Model file for the job. Use its own axes, mm. A direction names the side the tool comes from. Give positions to 0.01 mm unless a question says otherwise; leave off trailing zeros. Loops run counter-clockwise (first coordinate to the right, second up) from the corner with the lowest first, then second, coordinate; pieces in that order, holes last. Notation, with made-up numbers: M 1,-23.75 L 48,-23.75 A6 ccw 48,-12.75 Z; hole C 53.5,6.5 d3. An arc over 180 degrees is marked long. Use CSV: the item, a comma, the result in double quotes. Start each with the question number.
(1) Two-plate mould, pull along Y, no slides. Class faces 1 (the face through (8, 5.862, 0)), 2 (the face through (10.877, 10.2, 2.5)), 3 (the face through (3, 20, 3)), 4 (the face through (4, 10, -8.672)): pulls with the +Y half, pulls with the -Y half, needs draft (parallel to the pull), parting line crosses it, or undercut.
(2) Slice it at D-D on z = 34. List the corners of the cut face in (x, y), and give its area (3 significant figures).
(3) Flat gauge pins, fed straight in: P1, Ø0.6, axis at x = 3, z = 0, coming from the +Y side; P2, Ø5, axis at x = 7, y = 13.5, coming from the -Z side; P3, Ø9.5, axis at x = -7.5, z = 6, coming from the +Y side; P4, Ø6, axis at y = -3, z = 40, coming from the -X side. Where does each tip first touch, or does it go through?
(4) Slice it at C-C on z = -29. List the corners of the cut face in (x, y), and give its area (3 significant figures).
(5) Tool access for faces 5 (the face through (-3.4, 13.3, -0.1)), 6 (the face through (4, 10, 9.332)), 7 (the face through (8, 14.614, 0)): list every direction of +Z, -Z, +X, -X, +Y, -Y with a clear straight run to the whole face (end or side of a thin tool).
(6) Slice it at B-B on x = 0. List the corners of the cut face in (y, z).
(7) Wall check: line 1 along Z through (x, y) = (0, -7.5); line 2 along Z through (x, y) = (0, 16); line 3 along Y through (x, z) = (3, 0). Give the ranges that are in metal, low to high. Write a range as from..to.
(8) Slice it at A-A on y = -14.5. List the corners of the cut face in (x, z), and give its area (3 significant figures).
```python
from build123d import *

# Parameters (mm, degrees)
SKETCH1_R               = 6
BOSS_EXTRUDE1_DEPTH     = 20
SKETCH2_R               = 3.4
CUT_EXTRUDE1_DEPTH      = 13.55
SKETCH5_W               = 1.550685087
SKETCH5_H               = 7.184215806
BOSS_EXTRUDE2_DEPTH     = 13.55
SKETCH7_W               = 18.003976239
SKETCH7_H               = 19.909960041
BOSS_EXTRUDE3_DEPTH     = 10
SKETCH6_R               = 2
CUT_EXTRUDE2_DEPTH      = 1
CUT_EXTRUDE2_DEPTH_BACK = 13.55
CUT_EXTRUDE3_DEPTH      = 10
CUT_EXTRUDE3_DEPTH_BACK = 10
SKETCH10_R              = 50
BOSS_EXTRUDE4_DEPTH     = 30
SKETCH12_R              = 42.124366513
SKETCH12_R_2            = 15.95790089
CUT_EXTRUDE5_DEPTH      = 27


with BuildPart() as part:
    # Sketch1 → Boss-Extrude1 (new body)
    with BuildSketch(Plane(origin=(0, 0, 0), x_dir=(1, 0, 0), z_dir=(0, 1, 0))):
        Circle(SKETCH1_R)
    extrude(amount=BOSS_EXTRUDE1_DEPTH)

    # Sketch2 → Cut-Extrude1 (cut)
    with BuildSketch(Plane(origin=(0, 20, 0), x_dir=(1, 0, 0), z_dir=(0, 1, 0))):
        Circle(SKETCH2_R)
    extrude(amount=-CUT_EXTRUDE1_DEPTH, mode=Mode.SUBTRACT)

    # Sketch5 → Boss-Extrude2 (add)
    with BuildSketch(Plane(origin=(0, 18.26, 0), x_dir=(1, 0, 0), z_dir=(0, 1, 0))):
        with Locations((3.375342544, 0.020519704)):
            Rectangle(SKETCH5_W, SKETCH5_H)
    extrude(amount=-BOSS_EXTRUDE2_DEPTH)

    # Sketch7 → Boss-Extrude3 (add)
    with BuildSketch(Plane.ZY.offset(-2.6)):
        with Locations((0.33027221, 9.954980021)):
            Rectangle(SKETCH7_W, SKETCH7_H)
    extrude(amount=-BOSS_EXTRUDE3_DEPTH)

    # Sketch6 → Cut-Extrude2 (cut, two sides)
    with BuildSketch(Plane.ZY.offset(-2.6)) as cut_extrude2_sk:
        with Locations((0, 10.236925537)):
            Circle(SKETCH6_R)
    extrude(amount=CUT_EXTRUDE2_DEPTH, mode=Mode.SUBTRACT)
    extrude(cut_extrude2_sk.sketch, amount=-CUT_EXTRUDE2_DEPTH_BACK, mode=Mode.SUBTRACT)

    # Sketch9 → Cut-Extrude3 (cut, two sides)
    with BuildSketch(Plane.XY) as cut_extrude3_sk:
        Polygon((10.876516382, 10.236925537), (10.876516382, 5.861925537), (4.943430227, 5.861925537), (4.943430227, 10.236925537), (4.943430227, 14.614332445), (10.876516382, 14.614332445), align=None)
    extrude(amount=CUT_EXTRUDE3_DEPTH, mode=Mode.SUBTRACT)
    extrude(cut_extrude3_sk.sketch, amount=-CUT_EXTRUDE3_DEPTH_BACK, mode=Mode.SUBTRACT)

    # Sketch10 → Boss-Extrude4 (add)
    with BuildSketch(Plane.XZ):
        Circle(SKETCH10_R)
    extrude(amount=BOSS_EXTRUDE4_DEPTH)

    # Sketch12 → Cut-Extrude5 (cut)
    with BuildSketch(Plane(origin=(0, 0, 0), x_dir=(1, 0, 0), z_dir=(0, 1, 0))):
        Circle(SKETCH12_R)
        Circle(SKETCH12_R_2, mode=Mode.SUBTRACT)
    extrude(amount=-CUT_EXTRUDE5_DEPTH, mode=Mode.SUBTRACT)


solid = part.part
```
Reply:
1,face 1,"undercut"
1,face 2,"undercut"
1,face 3,"pulls with the +Y half"
1,face 4,"needs draft"
2,outline,"M -36.66,-30 L 36.66,-30 L 36.66,0 L 24.87,0 L 24.87,-27 L -24.87,-27 L -24.87,0 L -36.66,0 Z"
2,area,"857 mm^2"
3,P1,"stops at y = 19.91"
3,P2,"stops at z = -8.67"
3,P3,"stops at y = 20"
3,P4,"stops at x = -33.63"
4,outline,"M -40.73,-30 L 40.73,-30 L 40.73,0 L 30.55,0 L 30.55,-27 L -30.55,-27 L -30.55,0 L -40.73,0 Z"
4,area,"794 mm^2"
5,face 5,"+Y"
5,face 6,"+Z, +X, -X, +Y"
5,face 7,"+Z, -Z"
6,outline,"M -30,-50 L 0,-50 L 0,-42.12 L -27,-42.12 L -27,-15.96 L 0,-15.96 L 0,-6 L 20,-6 L 20,-3.4 L 6.45,-3.4 L 6.45,3.4 L 20,3.4 L 20,6 L 0,6 L 0,15.96 L -27,15.96 L -27,42.12 L 0,42.12 L 0,50 L -30,50 Z"
7,line 1,"z = -50..-42.12, -15.96..15.96, 42.12..50"
7,line 2,"z = -6..-3.4, 3.4..6"
7,line 3,"y = -30..8.24, 12.24..19.91"
8,outline,"C 0,0 d100; C 0,0 d31.92; hole C 0,0 d84.25"
8,area,"3,080 mm^2"
